Geometry check sheet. Reference: the model listing, model coordinates, mm. Face numbers are marked on the shaded views. A direction names the side the tool comes from. Give positions to 0.01 mm unless a question says otherwise; leave off trailing zeros. Write each loop counter-clockwise with the first axis right and the second up, starting at its lowest first coordinate (ties: lowest second). Pieces come first, ordered by that corner, then holes. Notation, with made-up numbers: M 27.5,44.5 L 79.5,44.5 A28 ccw 79.5,66.5 Z; hole C 36.25,3.25 d8. An arc over 180 degrees is marked long. One line per item, written item: value. Start each with the question number.
1. Scan lines: line 1 (X direction, y = 38, z = 32); line 2 (X direction, y = 48, z = 8); line 3 (X direction, y = 49.5, z = 22.5). Record each from-to range of solid material in increasing order.
2. Cross-section at D-D on y = 43. Record the cut outline in (x, z), then the cut area to 3 significant figures.
3. Release check for a two-part mould opening along X. For the marked faces 1, 2 and 3 record: pulls with the +X half, pulls with the -X half, needs draft (parallel to the pull), parting line crosses it, or undercut.
4. Cross-section at C-C on x = 11. Record the cut outline in (y, z), then the cut area to 3 significant figures.
5. Cross-section at A-A on z = 32. Record the cut outline in (x, y).
6. Tool access check on the marked faces 4, 5 and 6. Record the directions out of +Z, -Z, +X, -X, +Y, -Y that give a thin tool (end or side, any length) a straight path to the whole face; none if there is none.
7. Cross-section at B-B on x = 91. Record the cut outline in (y, z), then the cut area to 3 significant figures.
8. Gauge pin test, flat end, axial feed: pin 1 (9.5 mm diameter, centred on x = 11.5, z = 20.5, fed in from +Y). Record the tip position at first contact, or that the pin passes through.
from build123d import *

# Parameters (mm, degrees)
EXTRUDE_1_DEPTH     = 40
SKETCH_2_R          = 3.25
CUT_EXTRUDE_1_DEPTH = 126.39936204


with BuildPart() as part:
    # 草图1 → 凸台-拉伸1 (new body)
    with BuildSketch(Plane.XY):
        with BuildLine():
            Line((0, 61), (19, 61))
            Line((19, 61), (36, 78))
            Line((36, 78), (66, 78))
            Line((66, 78), (83, 61))
            Line((83, 61), (102, 61))
            Line((102, 61), (102, 41.5))
            Line((102, 41.5), (83.484611742, 41.5))
            ThreePointArc((83.484611742, 41.5), (18.5, 40.5), (83.484611742, 39.5))
            Line((83.484611742, 39.5), (102, 39.5))
            Line((102, 39.5), (102, 0))
            Line((102, 0), (0, 0))
            Line((0, 0), (0, 61))
        make_face()
    extrude(amount=EXTRUDE_1_DEPTH)

    # 草图2 → 切除-拉伸1 (cut, through all)
    with BuildSketch(Plane(origin=(0, 61, 0), x_dir=(1, 0, 0), z_dir=(0, 1, 0))):
        with Locations(Location((11, -8, 0), (0, 0, 270))):
            Circle(SKETCH_2_R)
        with Locations(Location((11, -32, 0), (0, 0, 270))):
            Circle(SKETCH_2_R)
        with Locations(Location((91, -8, 0), (0, 0, 270))):
            Circle(SKETCH_2_R)
        with Locations(Location((91, -32, 0), (0, 0, 270))):
            Circle(SKETCH_2_R)
    extrude(amount=-CUT_EXTRUDE_1_DEPTH, mode=Mode.SUBTRACT)


solid = part.part
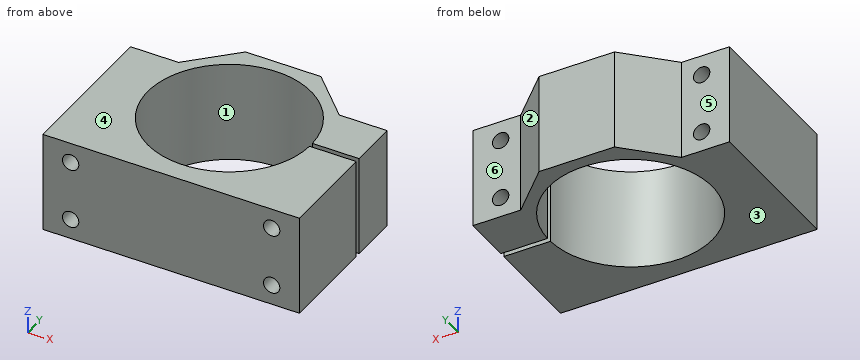
Report:
1. line 1: x = 0 to 7.75, 14.25 to 18.6, 83.4 to 87.75, 94.25 to 102
1. line 2: x = 0 to 7.75, 14.25 to 19.38, 82.62 to 87.75, 94.25 to 102
1. line 3: x = 0 to 19.77, 82.23 to 102
2. outline: M 0,0 L 18.6,0 L 18.6,40 L 0,40 Z; M 83.4,0 L 102,0 L 102,40 L 83.4,40 Z; hole C 11,8 d6.5; hole C 11,32 d6.5; hole C 91,8 d6.5; hole C 91,32 d6.5
2. area: 1,350 mm^2
3. face 1: undercut
3. face 2: pulls with the +X half
3. face 3: needs draft
4. outline: M 0,0 L 61,0 L 61,4.75 L 0,4.75 Z; M 0,11.25 L 61,11.25 L 61,28.75 L 0,28.75 Z; M 0,35.25 L 61,35.25 L 61,40 L 0,40 Z
4. area: 1,650 mm^2
5. outline: M 0,0 L 7.75,0 L 7.75,61 L 0,61 Z; M 14.25,0 L 87.75,0 L 87.75,39.5 L 83.48,39.5 A32.5 cw long 83.48,41.5 L 87.75,41.5 L 87.75,61 L 83,61 L 66,78 L 36,78 L 19,61 L 14.25,61 Z; M 94.25,0 L 102,0 L 102,39.5 L 94.25,39.5 Z; M 94.25,41.5 L 102,41.5 L 102,61 L 94.25,61 Z
6. face 4: +Z, +X, -X, +Y, -Y
6. face 5: +Z, -Z, -X, +Y
6. face 6: +Z, -Z, +X, +Y
7. outline: M 0,0 L 39.5,0 L 39.5,4.75 L 0,4.75 Z; M 0,11.25 L 39.5,11.25 L 39.5,28.75 L 0,28.75 Z; M 0,35.25 L 39.5,35.25 L 39.5,40 L 0,40 Z; M 41.5,0 L 61,0 L 61,4.75 L 41.5,4.75 Z; M 41.5,11.25 L 61,11.25 L 61,28.75 L 41.5,28.75 Z; M 41.5,35.25 L 61,35.25 L 61,40 L 41.5,40 Z
7. area: 1,590 mm^2
8. pin 1: stops at y = 61
